Build history of the part. All positions in model axes, mm. Face numbers are marked on the shaded views. A direction names the side the tool comes from. Round coordinates to 2 decimals unless told otherwise and drop trailing zeros. Write each loop counter-clockwise with the first axis right and the second up, starting at its lowest first coordinate (ties: lowest second). Pieces come first, ordered by that corner, then holes. Notation, with made-up numbers: (-1.5, 67.5) - (3.5, 67.5) arc R32 ccw to (3.5, 102.5) - close; hole circle Ø7 at (27, -15.5). An arc over 180 degrees is marked (long way). One line per question, with ' | ' between items.
from build123d import *

# Parameters (mm, degrees)
F2_DEPTH        = 2.15
F3_W            = 3
F3_H            = 7
F4_DEPTH        = 1.4
F5_SIZE2        = 1.39999
F5_SIZE         = 2.99999
F6_W            = 3
F6_H            = 2.55
F7_DEPTH        = 2.5
F8_W            = 43.1
F8_H            = 2.55
F9_DEPTH        = 3
F11_D           = 4
F11_CBORE_D     = 6.75
F11_CBORE_DEPTH = 5.5


# Not quite as in the source:
# - a fillet or chamfer is up to 0.001 mm smaller than in the source, because OpenCascade refuses the exact size


with BuildPart() as f2:
    # F1 (on Top) → F2 (new body)
    with BuildSketch(Plane.XY):
        Polygon((-23.05, -5), (-23.05, -10.05), (23.05, -10.05), (23.05, 10.05), (-23.05, 10.05), (-23.05, 5), (-9.05, 5), (-9.05, 3.5), (-23.05, 3.5), (-23.05, -3.5), (-9.05, -3.5), (-9.05, -5), align=None)
    extrude(amount=F2_DEPTH)

    # F3 (on face) → F4 (join)
    with BuildSketch(Plane.XY.offset(2.15)):
        with Locations((-19.55, 0)):
            Rectangle(F3_W, F3_H)
    extrude(amount=F4_DEPTH)

    # F5 (size 3 and 1.4 in the source; OpenCascade refuses exactly that, so slightly less here)
    f5_edges = [f2.edges().sort_by_distance(p)[0] for p in [
        (-21.05, 0, 3.55),
    ]]
    f5_side = f2.faces().sort_by_distance((-19.55, 0, 3.55))[0]
    chamfer(f5_edges, length=F5_SIZE, length2=F5_SIZE2, reference=f5_side)

    # F6 (on face) → F7 (join)
    with BuildSketch(Plane(origin=(0, 0, 0), x_dir=(1, 0, 0), z_dir=(0, 0, -1))):
        Polygon((-23.05, -5), (-23.05, -7.5), (20.05, -7.5), (23.05, -7.5), (23.05, 7.5), (20.05, 7.5), (-23.05, 7.5), (-23.05, 5), (-9.05, 5), (-9.05, 3.5), (-9.05, -3.5), (-9.05, -5), align=None)
        with Locations((21.55, 8.775)):
            Rectangle(F6_W, F6_H)
        with Locations((21.55, -8.775)):
            Rectangle(F6_W, F6_H)
    extrude(amount=F7_DEPTH)

    # F8 (on face) → F9 (join)
    with BuildSketch(Plane(origin=(0, 0, -2.5), x_dir=(1, 0, 0), z_dir=(0, 0, -1))):
        Polygon((23.05, -10.05), (23.05, 10.05), (20.05, 10.05), (20.05, 7.5), (-23.05, 7.5), (-23.05, 5), (-9.05, 5), (-9.05, -5), (-23.05, -5), (-23.05, -7.5), (20.05, -7.5), (20.05, -10.05), align=None)
        with Locations((-1.5, -8.775)):
            Rectangle(F8_W, F8_H)
        with Locations((-1.5, 8.775)):
            Rectangle(F8_W, F8_H)
    extrude(amount=F9_DEPTH)

    # F11 (through all)
    with Locations(Plane.XY.offset(2.15)):
        with Locations((1.05, 0)):
            CounterBoreHole(F11_D / 2, F11_CBORE_D / 2, F11_CBORE_DEPTH)


solid = f2.part
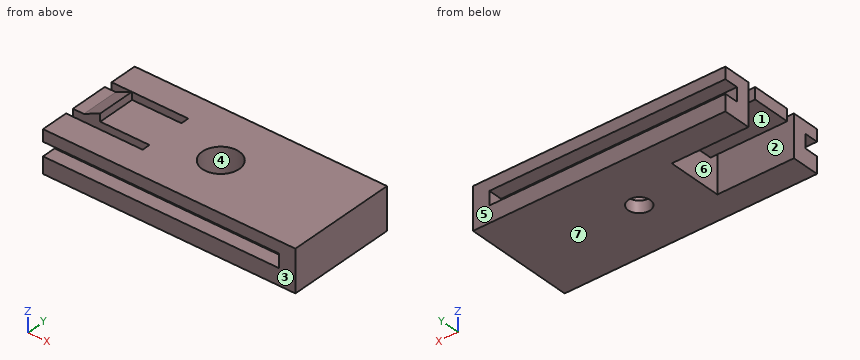
Q1. Drill centre lines: L1, parallel to Y at x = 1.05, z = -4.9; L2, parallel to Z at x = -6.5, y = -8.75; L3, parallel to Y at x = -13, z = -1.75. Where is each one in solid material? Low to high. Write a range as from..to.
Found:
L1: -10.05..-2, 2..10.05 | L2: -5.5..-2.5, 0..2.15 | L3: -7.5..-5, 5..7.5
Q2. Which spindle directions (+Z, -Z, +X, -X, +Y, -Y) get a long thin tool onto all of the face, cutting with end or side? Do the marked faces 1, 2, 3 and 4. Say none if no direction does.
Found:
face 1: -Z, -X | face 2: +Z, -Z, -X | face 3: +Z, -Z, +X, -X, -Y | face 4: +Z
Q3. Saw through at B-B, the plane x = -13. List the corners of the cut face in (y, z).
Found:
outline: (-10.05, -5.5) - (-5, -5.5) - (-5, 2.15) - (-10.05, 2.15) - (-10.05, 0) - (-7.5, 0) - (-7.5, -2.5) - (-10.05, -2.5) - close; (-3.5, 0) - (3.5, 0) - (3.5, 2.15) - (-3.5, 2.15) - close; (5, -5.5) - (10.05, -5.5) - (10.05, -2.5) - (7.5, -2.5) - (7.5, 0) - (10.05, 0) - (10.05, 2.15) - (5, 2.15) - close
Q4. Drop flat-ended pins along their axis: pin 1 (5 mm diameter, centred on x = 16.5, y = -5, fed in from +Z); pin 2 (1.1 mm diameter, centred on x = -17.5, z = 2.5, fed in from -Y); pin 3 (7.5 mm diameter, centred on x = -15, y = 1, fed in from -Z). Give the stop position or say it passes through.
Found:
pin 1: z = 2.15 | pin 2: y = -10.05 | pin 3: z = 0
Q5. Pull direction Y, two halves, no side cores. Call the marked faces 5, 6 and 7: +Y half, -Y half, draft (parallel to the pull), parting line (faces both ways), or undercut.
Found:
face 5: +Y half | face 6: undercut | face 7: draft
Q6. Saw through at C-C, the plane z = -0.5. List the corners of the cut face in (x, y) (3 decimals), then the cut area to 3 significant figures.
Found:
outline: (-23.05, -7.5) - (20.05, -7.5) - (20.05, -10.05) - (23.05, -10.05) - (23.05, 10.05) - (20.05, 10.05) - (20.05, 7.5) - (-23.05, 7.5) - (-23.05, 5) - (-9.05, 5) - (-9.05, -5) - (-23.05, -5) - close; hole circle Ø6.75 at (1.05, 0) | area: 531 mm^2
Q7. Saw through at D-D, the plane x = 1.05. List the corners of the cut face in (y, z) (3 decimals).
Found:
outline: (-10.05, -5.5) - (-2, -5.5) - (-2, -3.35) - (-3.375, -3.35) - (-3.375, 2.15) - (-10.05, 2.15) - (-10.05, 0) - (-7.5, 0) - (-7.5, -2.5) - (-10.05, -2.5) - close; (2, -5.5) - (10.05, -5.5) - (10.05, -2.5) - (7.5, -2.5) - (7.5, 0) - (10.05, 0) - (10.05, 2.15) - (3.375, 2.15) - (3.375, -3.35) - (2, -3.35) - close
